```python
from build123d import *

# Parameters (mm, degrees)
SKETCH1_R           = 15
BOSS_EXTRUDE3_DEPTH = 5


with BuildPart() as part:
    # Sketch1 → Boss-Extrude3 (new, symmetric)
    with BuildSketch(Plane.XY):
        with BuildLine():
            Line((0, 0), (0, 20))
            Line((0, 20), (35, 20))
            Line((35, 20), (35, 15))
            Line((35, 15), (60.563909774, 15))
            Line((60.563909774, 15), (60.563909774, 20))
            Line((60.563909774, 20), (90, 20))
            Line((90, 20), (90, 57.593984962))
            ThreePointArc((90, 57.593984962), (120, 87.593984962), (150, 57.593984962))
            Line((150, 57.593984962), (150, 0))
            Line((150, 0), (0, 0))
        make_face()
        with Locations((120, 57.593984962)):
            Circle(SKETCH1_R, mode=Mode.SUBTRACT)
    extrude(amount=BOSS_EXTRUDE3_DEPTH, both=True)


solid = part.part
```
The listing builds one solid part. Answer for the finished solid, in the listing's coordinates (mm). A direction names the side the tool comes from. Give positions to 0.01 mm unless a question says otherwise; leave off trailing zeros. Loops run counter-clockwise (first coordinate to the right, second up) from the corner with the lowest first, then second, coordinate; pieces in that order, holes last. Notation, with made-up numbers: (13.25, -20.75) - (32.25, -20.75) arc R25 ccw to (32.25, 16.25) - close; hole circle Ø2 at (38.5, 64.25). An arc over 180 degrees is marked (long way). Return JSON: item names as keys, results as strings. Group by question number.
1. Find section A-A (x = 120). Write down the section's boundary in (y, z), then the cut area to 3 significant figures.
2. Given pin 1 Ø3 at (y, z) = (32, 1) entering from -X; pin 2 Ø3 at (x, z) = (15.5, 0.5) entering from +Y, each flat-ended and moving along its own axis, determine where each tip first touches the part or whether it passes through.
3. Straight lines are drawn through the part: line 1 (Y direction, x = 120, z = 2); line 2 (X direction, y = 41, z = -1); line 3 (Y direction, x = 72, z = 2). For each, find the intervals that lie inside material, in ascending order. Write a range as [from, to].
4. Find section D-D (x = 49.5). Write down the section's boundary in (y, z), then the cut area to 3 significant figures.
5. Which of the six approach directions +Z, -Z, +X, -X, +Y, -Y give full straight-line access (tool end or side, diameter ignored) to faces 1 (the flat face through (90, 39, 0)), 2 (the flat face through (60.564, 17, 0)), 3 (the flat face through (150, 29, 0))?
6. Find section B-B (z = -0.5). Write down the section's boundary in (x, y), then the cut area to 3 significant figures.
7. Find section C-C (y = 56). Write down the section's boundary in (x, z), then the cut area to 3 significant figures.
Verdict:
{
 "1": {"outline": "(0, -5) - (42.59, -5) - (42.59, 5) - (0, 5) - close; (72.59, -5) - (87.59, -5) - (87.59, 5) - (72.59, 5) - close", "area": "576 mm^2"},
 "2": {"pin 1": "stops at x = 90", "pin 2": "stops at y = 20"},
 "3": {"line 1": "y = [0, 42.59], [72.59, 87.59]", "line 2": "x = [90, 150]", "line 3": "y = [0, 20]"},
 "4": {"outline": "(0, -5) - (15, -5) - (15, 5) - (0, 5) - close", "area": "150 mm^2"},
 "5": {"face 1": "+Z, -Z, -X, +Y", "face 2": "+Z, -Z, +Y", "face 3": "+Z, -Z, +X, +Y, -Y"},
 "6": {"outline": "(0, 0) - (150, 0) - (150, 57.59) arc R30 ccw to (90, 57.59) - (90, 20) - (60.56, 20) - (60.56, 15) - (35, 15) - (35, 20) - (0, 20) - close; hole circle Ø30 at (120, 57.59)", "area": "5,830 mm^2"},
 "7": {"outline": "(90, -5) - (105.08, -5) - (105.08, 5) - (90, 5) - close; (134.92, -5) - (150, -5) - (150, 5) - (134.92, 5) - close", "area": "302 mm^2"}
}
